Verification items for the finished model (mm, model axes). Face numbers are marked on the shaded views. Round coordinates to 2 decimals unless told otherwise and drop trailing zeros. Loops run counter-clockwise (first coordinate to the right, second up) from the corner with the lowest first, then second, coordinate; pieces in that order, holes last. Notation, with made-up numbers: (-27.5, 62) -> (-1.5, 62) arc R10 cw to (-1.5, 77) -> close; hole circle Ø10 at (8, 30.5). An arc over 180 degrees is marked (long way). Write item = value, one per line.
```python
from build123d import *

# Parameters (mm, degrees)
SKETCH1_W      = 65
SKETCH1_H      = 65
EXTRUDE1_DEPTH = 3
CHAMFER1_SIZE  = 8.125
EXTRUDE2_DEPTH = 5
SKETCH3_W      = 12
SKETCH3_H      = 35
EXTRUDE3_DEPTH = 3
SKETCH4_R      = 2.3
EXTRUDE4_DEPTH = 3


with BuildPart() as part:
    # Sketch1 → Extrude1 (new body)
    with BuildSketch(Plane(origin=(0, 0, 0), x_dir=(1, 0, 0), z_dir=(0, 1, 0))):
        Rectangle(SKETCH1_W, SKETCH1_H)
    extrude(amount=EXTRUDE1_DEPTH)

    # Chamfer1
    chamfer1_edges = [part.edges().sort_by_distance(p)[0] for p in [
        (32.5, 1.5, 32.5),
        (-32.5, 1.5, 32.5),
        (-32.5, 1.5, -32.5),
        (32.5, 1.5, -32.5),
    ]]
    chamfer(chamfer1_edges, length=CHAMFER1_SIZE)

    # Sketch2 → Extrude2 (add)
    with BuildSketch(Plane(origin=(0, 3, 0), x_dir=(1, 0, 0), z_dir=(0, 1, 0))):
        Polygon((22.552460326, 28.1), (-22.552460326, 28.1), (-28.1, 22.552460326), (-28.1, -22.552460326), (-22.552460326, -28.1), (22.552460326, -28.1), (28.1, -22.552460326), (28.1, 22.552460326), align=None)
        Polygon((-21.724033201, 26.1), (-26.1, 21.724033201), (-26.1, -11.272604381), (-26.1, -21.724033201), (-21.724033201, -26.1), (21.724033201, -26.1), (26.1, -21.724033201), (26.1, 21.724033201), (21.724033201, 26.1), align=None, mode=Mode.SUBTRACT)
    extrude(amount=EXTRUDE2_DEPTH)

    # Sketch3 → Extrude3 (add)
    with BuildSketch(Plane(origin=(0, 3, 0), x_dir=(1, 0, 0), z_dir=(0, 1, 0))):
        with Locations((-13.296722284, 0)):
            Rectangle(SKETCH3_W, SKETCH3_H)
    extrude3 = extrude(amount=EXTRUDE3_DEPTH)

    # Mirror1: Extrude3 across plane
    add(extrude3.mirror(Plane(origin=(0, 0, 0), x_dir=(0, 0, 1), z_dir=(1, 0, 0))))

    # Sketch4 → Extrude4 (cut)
    with BuildSketch(Plane(origin=(0, 3, 0), x_dir=(1, 0, 0), z_dir=(0, 1, 0))):
        with Locations(Location((0, 15, 0), (0, 0, 270))):
            Circle(SKETCH4_R)
        with Locations(Location((0, -15, 0), (0, 0, 270))):
            Circle(SKETCH4_R)
    extrude(amount=-EXTRUDE4_DEPTH, mode=Mode.SUBTRACT)


solid = part.part
```
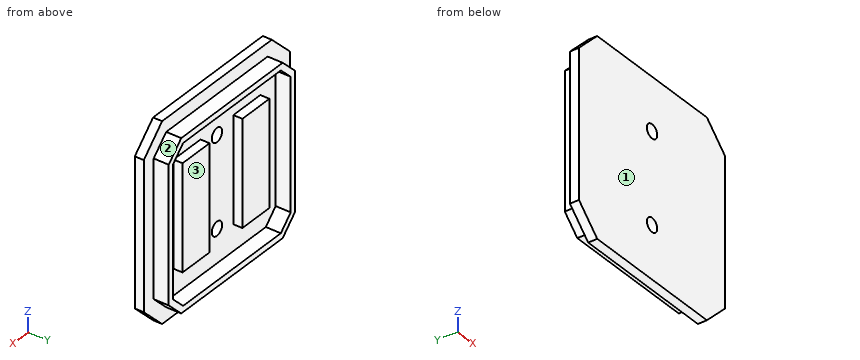
(1) Go/stop test with flat-tipped pins: pin 1 Ø4 at (y, z) = (6.5, -2) entering from +X; pin 2 Ø10 at (x, z) = (-4.5, 2) entering from +Y; pin 3 Ø2.5 at (x, y) = (-9.5, 4.5) entering from -Z; pin 4 Ø2.5 at (x, y) = (-14, 4) entering from -Z. Record where each tip stops, or that it passes through.
Filled sheet:
pin_1 = 28.1
pin_2 = 6
pin_3 = -28.1
pin_4 = -32.5
(2) Sectioned sample at D-D, the plane x = -14. Record the cut outline in (y, z), and give its area (3 significant figures).
Filled sheet:
outline = (0, -32.5) -> (3, -32.5) -> (3, -28.1) -> (8, -28.1) -> (8, -26.1) -> (3, -26.1) -> (3, -17.5) -> (6, -17.5) -> (6, 17.5) -> (3, 17.5) -> (3, 26.1) -> (8, 26.1) -> (8, 28.1) -> (3, 28.1) -> (3, 32.5) -> (0, 32.5) -> close
area = 320 mm2
(3) Sectioned sample at C-C, the plane y = 4.5. Record the cut outline in (x, z).
Filled sheet:
outline = (-28.1, -22.55) -> (-22.55, -28.1) -> (22.55, -28.1) -> (28.1, -22.55) -> (28.1, 22.55) -> (22.55, 28.1) -> (-22.55, 28.1) -> (-28.1, 22.55) -> close; (-19.3, -17.5) -> (-7.3, -17.5) -> (-7.3, 17.5) -> (-19.3, 17.5) -> close; (7.3, -17.5) -> (19.3, -17.5) -> (19.3, 17.5) -> (7.3, 17.5) -> close; hole (-26.1, -21.72) -> (-21.72, -26.1) -> (21.72, -26.1) -> (26.1, -21.72) -> (26.1, 21.72) -> (21.72, 26.1) -> (-21.72, 26.1) -> (-26.1, 21.72) -> close
(4) Material ranges on probe 1 along X at (y, z) = (6.5, -8.5); probe 2 along X at (y, z) = (4, -3), recorded low to high. Write a range as from..to.
Filled sheet:
probe_1 = -28.1..-26.1, 26.1..28.1
probe_2 = -28.1..-26.1, -19.3..-7.3, 7.3..19.3, 26.1..28.1
(5) Sectioned sample at A-A, the plane z = 15. Record the cut outline in (x, y), and give its area (3 significant figures).
Filled sheet:
outline = (-32.5, 0) -> (-2.3, 0) -> (-2.3, 3) -> (-7.3, 3) -> (-7.3, 6) -> (-19.3, 6) -> (-19.3, 3) -> (-26.1, 3) -> (-26.1, 8) -> (-28.1, 8) -> (-28.1, 3) -> (-32.5, 3) -> close; (2.3, 0) -> (32.5, 0) -> (32.5, 3) -> (28.1, 3) -> (28.1, 8) -> (26.1, 8) -> (26.1, 3) -> (19.3, 3) -> (19.3, 6) -> (7.3, 6) -> (7.3, 3) -> (2.3, 3) -> close
area = 273 mm2
(6) Sectioned sample at B-B, the plane x = 0. Record the cut outline in (y, z).
Filled sheet:
outline = (0, -32.5) -> (3, -32.5) -> (3, -28.1) -> (8, -28.1) -> (8, -26.1) -> (3, -26.1) -> (3, -17.3) -> (0, -17.3) -> close; (0, -12.7) -> (3, -12.7) -> (3, 12.7) -> (0, 12.7) -> close; (0, 17.3) -> (3, 17.3) -> (3, 26.1) -> (8, 26.1) -> (8, 28.1) -> (3, 28.1) -> (3, 32.5) -> (0, 32.5) -> close
(7) Draft check along X on the marked faces 1, 2 and 3. Enter one of: released by +X, released by -X, zero draft, split by the parting line, or undercut.
Filled sheet:
face_1 = zero draft
face_2 = released by +X
face_3 = undercut
